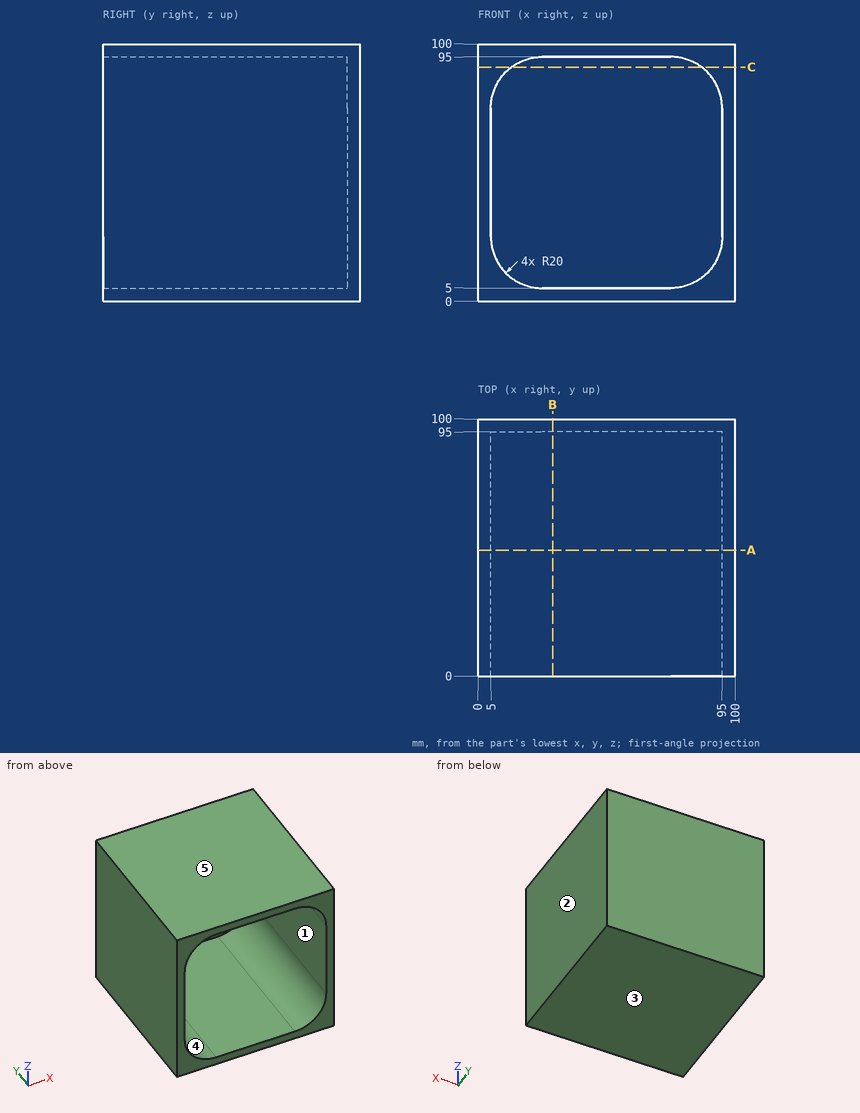
Check sheet for the drawn part. Datum: minimum x, y, z corner. Units: mm. A direction names the side the tool comes from. Round coordinates to 2 decimals unless told otherwise and drop trailing zeros. Loops run counter-clockwise (first coordinate to the right, second up) from the corner with the lowest first, then second, coordinate; pieces in that order, holes last. Notation, with made-up numbers: (-15.75, -1.75) - (10.25, -1.75) arc R26 cw to (10.25, 37.25) - close; hole circle Ø9 at (-23, -6.5). An arc over 180 degrees is marked (long way). Write each question's results on one line, items separated by ' | '. Start each with the question number.
Q1. Cross-section at B-B on x = 29. Enter the section's corners in (y, z).
Q2. Cross-section at C-C on z = 91. Enter the section's corners in (x, y), and give its area (3 significant figures).
Q3. Cross-section at A-A on y = 49. Enter the section's corners in (x, z), and give its area (3 significant figures).
Q4. Access from +Z, -Z, +X, -X, +Y, -Y to the whole of each face (thin tool, end or side, straight path). Record for the marked faces 4 and 5.
Q5. Thickness scan on line 1 (Z direction, x = 55.5, y = 16); line 2 (Y direction, x = 70, z = 39). Record the ranges inside material, lowest first. Write a range as [from, to].
Q6. Release check for a two-part mould opening along X. For the marked faces 1, 2 and 3 record: +X half, -X half, draft (parallel to the pull), parting line (faces both ways), or undercut.
Answers below:
1) outline: (0, 0) - (100, 0) - (100, 100) - (0, 100) - (0, 95) - (95, 95) - (95, 5) - (0, 5) - close
2) outline: (0, 0) - (13, 0) - (13, 95) - (87, 95) - (87, 0) - (100, 0) - (100, 100) - (0, 100) - close | area: 2,970 mm²
3) outline: (0, 0) - (100, 0) - (100, 100) - (0, 100) - close; hole (5, 25) arc R20 ccw to (25, 5) - (75, 5) arc R20 ccw to (95, 25) - (95, 75) arc R20 ccw to (75, 95) - (25, 95) arc R20 ccw to (5, 75) - close | area: 2,240 mm²
4) face 4: -Y | face 5: +Z, +X, -X, +Y, -Y
5) line 1: z = [0, 5], [95, 100] | line 2: y = [95, 100]
6) face 1: undercut | face 2: +X half | face 3: draft
